Verification items for this drawing (mm, ordinates from the low corner). A direction names the side the tool comes from. Round coordinates to 2 decimals unless told otherwise and drop trailing zeros. Loops run counter-clockwise (first coordinate to the right, second up) from the corner with the lowest first, then second, coordinate; pieces in that order, holes last. Notation, with made-up numbers: M -24.5,52 L 7.5,52 A24 cw 7.5,90 Z; hole C 54,-13 d7. An arc over 180 degrees is marked long. Write item = value, one per line. Start each with the question number.
(1) Cross-section at B-B on x = 7.23. Record the boundary of the cut face in (y, z), plus the area to 3 significant figures.
(2) Cross-section at A-A on y = 5.5. Record the boundary of the cut face in (x, z), plus the area to 3 significant figures.
(3) Go/stop test with flat-tipped pins: P1, Ø0.7, axis at y = 23.5, z = 3, coming from the +X side; P2, Ø4, axis at x = 2.5, y = 13.5, coming from the +Z side; P3, Ø1.2, axis at y = 24.5, z = 3, coming from the -X side. Record where each tip stops, or that it passes through.
(4) Mould release check, pull along X, two halves, no side actions. Record for the marked faces 1, 2 and 3: pulls with the +X half, pulls with the -X half, needs draft (parallel to the pull), parting line crosses it, or undercut.
(5) Scan lines: L1, parallel to Y at x = 15, z = 0.65; L2, parallel to Y at x = 9.77, z = 0.5; L3, parallel to Y at x = 6, z = 1.35. Record each from-to range of solid material in increasing order. Write a range as from..to.
(6) Cross-section at C-C on x = 15. Record the boundary of the cut face in (y, z).
(7) Set-up check for the marked faces 4, 5 and 6: record each of +Z, -Z, +X, -X, +Y, -Y from which the full face is reachable in a straight line by a thin tool's end or side.
(8) Cross-section at D-D on z = 0.8. State how many separate pieces and enclosed holes the cut face has, plus the area to 3 significant figures.
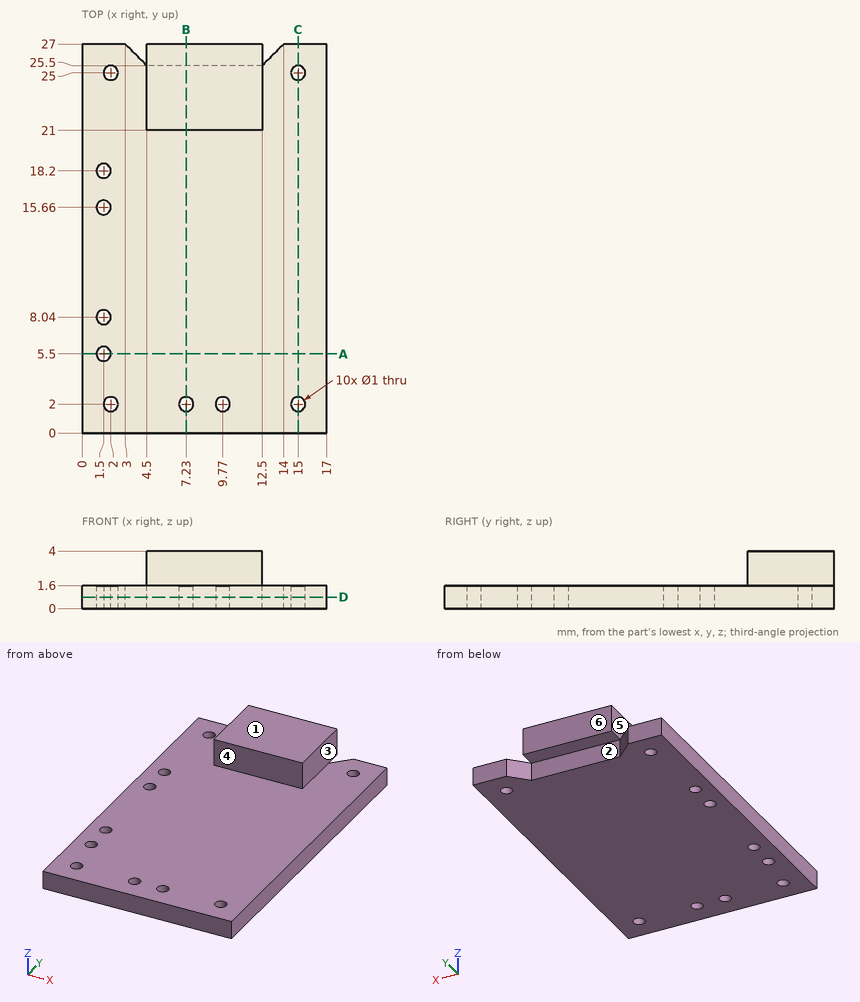
Result:
q1.outline = M 0,0 L 1.5,0 L 1.5,1.6 L 0,1.6 Z; M 2.5,0 L 25.5,0 L 25.5,1.6 L 27,1.6 L 27,4 L 21,4 L 21,1.6 L 2.5,1.6 Z
q1.area = 53.6 mm^2
q2.outline = M 0,0 L 1,0 L 1,1.6 L 0,1.6 Z; M 2,0 L 17,0 L 17,1.6 L 2,1.6 Z
q2.area = 25.6 mm^2
q3.P1 = 12.5
q3.P2 = 1.6
q3.P3 = 4.5
q4.face_1 = needs draft
q4.face_2 = undercut
q4.face_3 = pulls with the +X half
q5.L1 = 0..1.5, 2.5..24.5, 25.5..27
q5.L2 = 0..1.5, 2.5..25.5
q5.L3 = 0..25.5
q6.outline = M 0,0 L 1.5,0 L 1.5,1.6 L 0,1.6 Z; M 2.5,0 L 24.5,0 L 24.5,1.6 L 2.5,1.6 Z; M 25.5,0 L 27,0 L 27,1.6 L 25.5,1.6 Z
q7.face_4 = +Z, +X, -X, -Y
q7.face_5 = +Z, -X, +Y, -Y
q7.face_6 = +Z, -Z, +X, -X, +Y
q8.separate_pieces = 1
q8.enclosed_holes = 10
q8.area = 437 mm^2
